The listing builds one solid part. Answer for the finished solid, in the listing's coordinates (mm). Face numbers are marked on the shaded views. A direction names the side the tool comes from. Coordinates: 2 decimals unless noted, no trailing zeros. Order: outer loops, then holes, each group sorted by start corner. A loop starts at its lowest first (then second) coordinate and runs counter-clockwise, first axis right, second up.
```python
from build123d import *

# Parameters (mm, degrees)
SKETCH1_R           = 40
SKETCH1_R_2         = 21.5
BOSS_EXTRUDE1_DEPTH = 37.4
SKETCH1_3_R         = 21.5
BOSS_EXTRUDE2_DEPTH = 20.7
SKETCH1_5_R         = 1.5
BOSS_EXTRUDE3_DEPTH = 10.45


with BuildPart() as part:
    # Sketch1 → Boss-Extrude1 (new body)
    with BuildSketch(Plane(origin=(0, 0, 0), x_dir=(0, 0, -1), z_dir=(1, 0, 0))):
        Circle(SKETCH1_R)
        Circle(SKETCH1_R_2, mode=Mode.SUBTRACT)
    extrude(amount=BOSS_EXTRUDE1_DEPTH)

    # Sketch1_3 → Boss-Extrude2 (add)
    with BuildSketch(Plane(origin=(0, 0, 0), x_dir=(0, 0, -1), z_dir=(1, 0, 0))):
        Circle(SKETCH1_3_R)
        Polygon((1.905, -3.299556788), (3.81, 0), (1.905, 3.299556788), (-1.905, 3.299556788), (-3.81, 0), (-1.905, -3.299556788), align=None, mode=Mode.SUBTRACT)
    extrude(amount=BOSS_EXTRUDE2_DEPTH)

    # Sketch1_5 → Boss-Extrude3 (add)
    with BuildSketch(Plane(origin=(0, 0, 0), x_dir=(0, 0, -1), z_dir=(1, 0, 0))):
        Polygon((-1.905, -3.299556788), (1.905, -3.299556788), (3.81, 0), (1.905, 3.299556788), (-1.905, 3.299556788), (-3.81, 0), align=None)
        Circle(SKETCH1_5_R, mode=Mode.SUBTRACT)
    extrude(amount=BOSS_EXTRUDE3_DEPTH)


solid = part.part
```
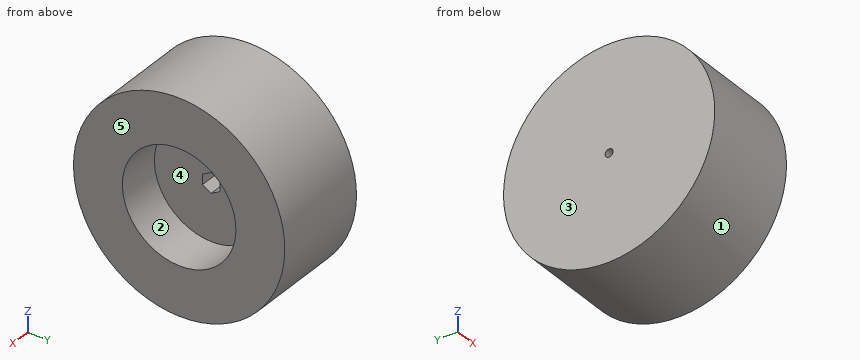
(1) Find section A-A (z = 0). Write down the section's boundary in (x, y).
(2) Consider line 1 (Y direction, x = 6, z = 0); line 2 (Y direction, x = 25, z = 0); line 3 (Z direction, x = 32, y = -26). Determine where each line is inside the solid, lowest interval first.
(3) For the marked faces 4 and 5, determine the directions among +Z, -Z, +X, -X, +Y, -Y from which every point of the face is accessible in a straight line to the end or side of a thin tool.
(4) Find section D-D (z = 15). Write down the section's boundary in (x, y).
(5) Find section C-C (y = 4.5). Write down the section's boundary in (x, z), and give its area (3 significant figures).
(6) Each of these flat-tipped pins is pushed along its axis until it touches: pin 1 Ø3 at (x, y) = (15, 7) entering from -Z; pin 2 Ø1 at (x, z) = (27, 18) entering from -Y; pin 3 Ø10 at (x, z) = (5, -6.5) entering from +Y; pin 4 Ø4 at (y, z) = (13.5, 5.5) entering from -X. Where does it stop, or does it pass through?
(7) Find section B-B (x = 17.5). Write down the section's boundary in (y, z) (3 decimals), and give its area (3 significant figures).
(8) The mould has two halves that part along Y. Classify the marked faces 1, 2 and 3: released by +Y, released by -Y, zero draft, split by the parting line, or undercut.
Findings below:
1. outline: (0, -40) - (37.4, -40) - (37.4, -21.5) - (20.7, -21.5) - (20.7, -3.3) - (10.45, -3.3) - (10.45, -1.5) - (0, -1.5) - close; (0, 1.5) - (10.45, 1.5) - (10.45, 3.3) - (20.7, 3.3) - (20.7, 21.5) - (37.4, 21.5) - (37.4, 40) - (0, 40) - close
2. line 1: y = -40 to -1.5, 1.5 to 40
2. line 2: y = -40 to -21.5, 21.5 to 40
2. line 3: z = -30.4 to 30.4
3. face 4: +X
3. face 5: +Z, -Z, +X, +Y, -Y
4. outline: (0, -37.08) - (37.4, -37.08) - (37.4, -15.4) - (20.7, -15.4) - (20.7, 15.4) - (37.4, 15.4) - (37.4, 37.08) - (0, 37.08) - close
5. outline: (0, -39.75) - (37.4, -39.75) - (37.4, -21.02) - (20.7, -21.02) - (20.7, 21.02) - (37.4, 21.02) - (37.4, 39.75) - (0, 39.75) - close
5. area: 2,270 mm2
6. pin 1: stops at z = -39.62
6. pin 2: stops at y = -35.97
6. pin 3: stops at y = 39.97
6. pin 4: stops at x = 0
7. outline: circle Ø80 at (0, 0); hole (-3.3, -1.905) - (0, -3.81) - (3.3, -1.905) - (3.3, 1.905) - (0, 3.81) - (-3.3, 1.905) - close
7. area: 4,990 mm2
8. face 1: split by the parting line
8. face 2: undercut
8. face 3: zero draft
